Geometry check sheet. Reference: the model listing, model coordinates, mm. A direction names the side the tool comes from. Coordinates: 2 decimals unless noted, no trailing zeros. Loops run counter-clockwise (first coordinate to the right, second up) from the corner with the lowest first, then second, coordinate; pieces in that order, holes last.
from build123d import *

# Parameters (mm, degrees)
F0_W     = 25.0952
F0_H     = 12.192
F1_DEPTH = 66.8274
F2_R     = 2.0193
F3_DEPTH = 25.4
F4_R     = 2.0193
F5_DEPTH = 19.05
F6_SIZE  = 1.778
F7_R     = 4.7625
F8_DEPTH = 12.193


with BuildPart() as f1:
    # F0 (on Front) → F1 (new body)
    with BuildSketch(Plane.XZ):
        Rectangle(F0_W, F0_H)
    extrude(amount=F1_DEPTH)

    # F2 (on face) → F3 (cut)
    with BuildSketch(Plane(origin=(0, 0, 0), x_dir=(-1, 0, 0), z_dir=(0, 1, 0))):
        with Locations((6.35, 0)):
            Circle(F2_R)
        with Locations((-6.35, 0)):
            Circle(F2_R)
    extrude(amount=-F3_DEPTH, mode=Mode.SUBTRACT)

    # F4 (on face) → F5 (cut)
    with BuildSketch(Plane.XZ.offset(66.8274)):
        with Locations((-4.9276, -1.8288)):
            Circle(F4_R)
        with Locations((4.9276, -1.8288)):
            Circle(F4_R)
    extrude(amount=-F5_DEPTH, mode=Mode.SUBTRACT)

    # F6
    f6_edges = [f1.edges().sort_by_distance(p)[0] for p in [
        (0, -66.8274, -6.096),
    ]]
    chamfer(f6_edges, length=F6_SIZE)

    # F7 (on face) → F8 (cut, through all)
    with BuildSketch(Plane(origin=(0, 0, -6.096), x_dir=(1, 0, 0), z_dir=(0, 0, -1))):
        with Locations((0, 42.6974)):
            Circle(F7_R)
    extrude(amount=-F8_DEPTH, mode=Mode.SUBTRACT)


solid = f1.part
(1) Sectioned sample at D-D on x = 3.75. Record the cut outline in (y, z).
Findings:
outline: (-66.83, -4.32) - (-65.05, -6.1) - (-45.63, -6.1) - (-45.63, 6.1) - (-66.83, 6.1) - (-66.83, -0.19) - (-47.78, -0.19) - (-47.78, -3.47) - (-66.83, -3.47) - close; (-39.76, -6.1) - (0, -6.1) - (0, 6.1) - (-39.76, 6.1) - close
(2) Sectioned sample at A-A on x = 0. Record the cut outline in (y, z).
Findings:
outline: (-66.83, -4.32) - (-65.05, -6.1) - (-47.46, -6.1) - (-47.46, 6.1) - (-66.83, 6.1) - close; (-37.93, -6.1) - (0, -6.1) - (0, 6.1) - (-37.93, 6.1) - close
(3) Scan lines: L1, parallel to Z at x = -6.35, y = -17.5; L2, parallel to Y at x = 0, z = 3; L3, parallel to X at y = -12, z = 0.25. Record each from-to range of solid material in increasing order.
Findings:
L1: z = -6.1 to -2.02, 2.02 to 6.1
L2: y = -66.83 to -47.46, -37.93 to 0
L3: x = -12.55 to -8.35, -4.35 to 4.35, 8.35 to 12.55
(4) Access from +Z, -Z, +X, -X, +Y, -Y to the whole of each face (thin tool, end or side, straight path). Record for faces 4 (the flat face through (-6, -25.4, 0)), 5 (the flat face through (0, 0, 0)), 6 (the flat face through (5, -47.777, -2)).
Findings:
face 4: +Y
face 5: +Z, -Z, +X, -X, +Y
face 6: -Y
(5) Gauge pin test, flat ends, axial feed: pin 1 Ø2 at (x, z) = (-5.5, -1.5) entering from -Y; pin 2 Ø1.2 at (x, z) = (5.5, -0.5) entering from +Y. Record the tip position at first contact, or that the pin passes through.
Findings:
pin 1: stops at y = -47.78
pin 2: stops at y = -25.4
(6) Sectioned sample at C-C on y = -23. Record the cut outline in (x, z).
Findings:
outline: (-12.55, -6.1) - (12.55, -6.1) - (12.55, 6.1) - (-12.55, 6.1) - close; hole circle Ø4.04 at (-6.35, 0); hole circle Ø4.04 at (6.35, 0)
(7) Sectioned sample at B-B on z = 1. Record the cut outline in (x, y) (1 decimal).
Findings:
outline: (-12.5, -66.8) - (12.5, -66.8) - (12.5, 0) - (8.1, 0) - (8.1, -25.4) - (4.6, -25.4) - (4.6, 0) - (-4.6, 0) - (-4.6, -25.4) - (-8.1, -25.4) - (-8.1, 0) - (-12.5, 0) - close; hole circle Ø9.5 at (0, -42.7)
(8) Draft check along Z on faces 1 (the cylindrical face through (-8.276, -12.522, 0.607)), 2 (the flat face through (0, -66.827, 1)), 3 (the flat face through (-0.176, -65.951, -5.195)). Enter one of: +Z half, -Z half, draft (parallel to the pull), parting line (faces both ways), or undercut.
Findings:
face 1: undercut
face 2: draft
face 3: -Z half
